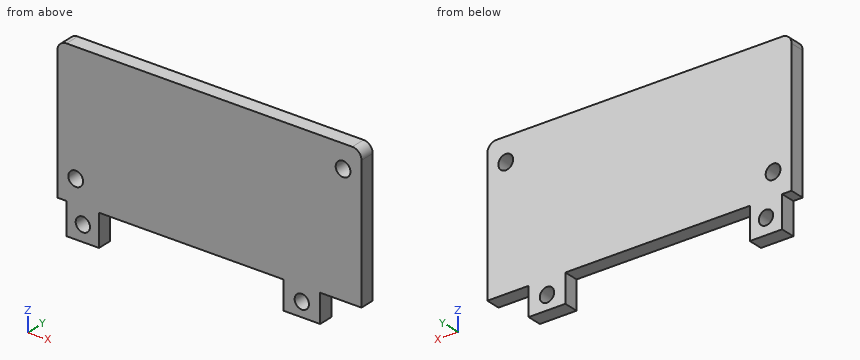
```python
from build123d import *

# Parameters (mm, degrees)
SKETCH2_R           = 1.6
SKETCH2_R_2         = 1.550000008
SKETCH2_R_3         = 1.55
BOSS_EXTRUDE1_DEPTH = 3.175
FILLET1_R           = 2


with BuildPart() as part:
    # Sketch2 → Boss-Extrude1 (new body)
    with BuildSketch(Plane(origin=(0, 0, 0), x_dir=(1, 0, 0), z_dir=(0, 1, 0))):
        Polygon((9.058586069, 30.8), (9.058586069, 37.689356794), (2.033404749, 37.689356794), (2.033404749, 30.8), (0, 30.8), (0, 0), (66, 0), (66, 30.8), (57.033404749, 30.8), (57.033404749, 36.920267815), (49.058586069, 36.920267815), (49.058586069, 30.8), align=None)
        with Locations(Location((62, 5, 0), (0, 0, 270))):
            Circle(SKETCH2_R, mode=Mode.SUBTRACT)
        with Locations(Location((4, 25.8, 0), (0, 0, 270))):
            Circle(SKETCH2_R, mode=Mode.SUBTRACT)
        with Locations(Location((5.545995409, 34.244678397, 0), (0, 0, 270))):
            Circle(SKETCH2_R_2, mode=Mode.SUBTRACT)
        with Locations(Location((53.045995409, 33.860133908, 0), (0, 0, 270))):
            Circle(SKETCH2_R_3, mode=Mode.SUBTRACT)
    extrude(amount=BOSS_EXTRUDE1_DEPTH)

    # Fillet1
    fillet1_edges = [part.edges().sort_by_distance(p)[0] for p in [
        (66, 1.5875, 0),
        (0, 1.5875, 0),
    ]]
    fillet(fillet1_edges, radius=FILLET1_R)


solid = part.part
```
Here's how the part is built. I have some questions about the finished solid (model axes, mm). Coordinates: 2 decimals unless noted, no trailing zeros. Loops run counter-clockwise (first coordinate to the right, second up) from the corner with the lowest first, then second, coordinate; pieces in that order, holes last. Notation, with made-up numbers: M 73.25,68 L 131.25,68 A7 cw 131.25,80 Z; hole C 35,-32 d2. An arc over 180 degrees is marked long. One line per item, written item: value.
1. Please list where these lines run through material, in increasing order: probe 1 along X at (y, z) = (2.3, -25.8); probe 2 along X at (y, z) = (0.8, -35); probe 3 along Z at (x, y) = (12.5, 1.4).
Geometry says:
probe 1: x = 0 to 2.4, 5.6 to 66
probe 2: x = 2.03 to 4.19, 6.9 to 9.06, 49.06 to 52, 54.1 to 57.03
probe 3: z = -30.8 to 0
2. Imagine slicing it at B-B (z = -5). List the corners of the cut face in (x, y) for me (3 decimals), and give its area (3 significant figures).
Geometry says:
outline: M 0,0 L 60.4,0 L 60.4,3.175 L 0,3.175 Z; M 63.6,0 L 66,0 L 66,3.175 L 63.6,3.175 Z
area: 199 mm2
3. Imagine slicing it at A-A (x = 62). List the corners of the cut face in (y, z) for me (3 decimals), and give its area (3 significant figures).
Geometry says:
outline: M 0,-30.8 L 3.175,-30.8 L 3.175,-6.6 L 0,-6.6 Z; M 0,-3.4 L 3.175,-3.4 L 3.175,0 L 0,0 Z
area: 87.6 mm2
4. Will these pins go through, and if not, where does the flat tip stop? pin 1 Ø1 at (y, z) = (1, -32) entering from +X; pin 2 Ø1 at (x, y) = (53, 1.5) entering from -Z; pin 3 Ø1.6 at (x, y) = (60, 1) entering from -Z.
Geometry says:
pin 1: stops at x = 57.03
pin 2: stops at z = -36.92
pin 3: stops at z = -30.8
5. Imagine slicing it at C-C (y = 2.2). List the corners of the cut face in (x, z) for me, and give its area (3 significant figures).
Geometry says:
outline: M 0,-30.8 L 2.03,-30.8 L 2.03,-37.69 L 9.06,-37.69 L 9.06,-30.8 L 49.06,-30.8 L 49.06,-36.92 L 57.03,-36.92 L 57.03,-30.8 L 66,-30.8 L 66,-2 A2 ccw 64,0 L 2,0 A2 ccw 0,-2 Z; hole C 4,-25.8 d3.2; hole C 5.55,-34.24 d3.1; hole C 53.05,-33.86 d3.1; hole C 62,-5 d3.2
area: 2,100 mm2
6. Imagine slicing it at D-D (z = -33.5). List the corners of the cut face in (x, y) for me (3 decimals), and give its area (3 significant figures).
Geometry says:
outline: M 2.033,0 L 4.187,0 L 4.187,3.175 L 2.033,3.175 Z; M 6.905,0 L 9.059,0 L 9.059,3.175 L 6.905,3.175 Z; M 49.059,0 L 51.538,0 L 51.538,3.175 L 49.059,3.175 Z; M 54.554,0 L 57.033,0 L 57.033,3.175 L 54.554,3.175 Z
area: 29.4 mm2
